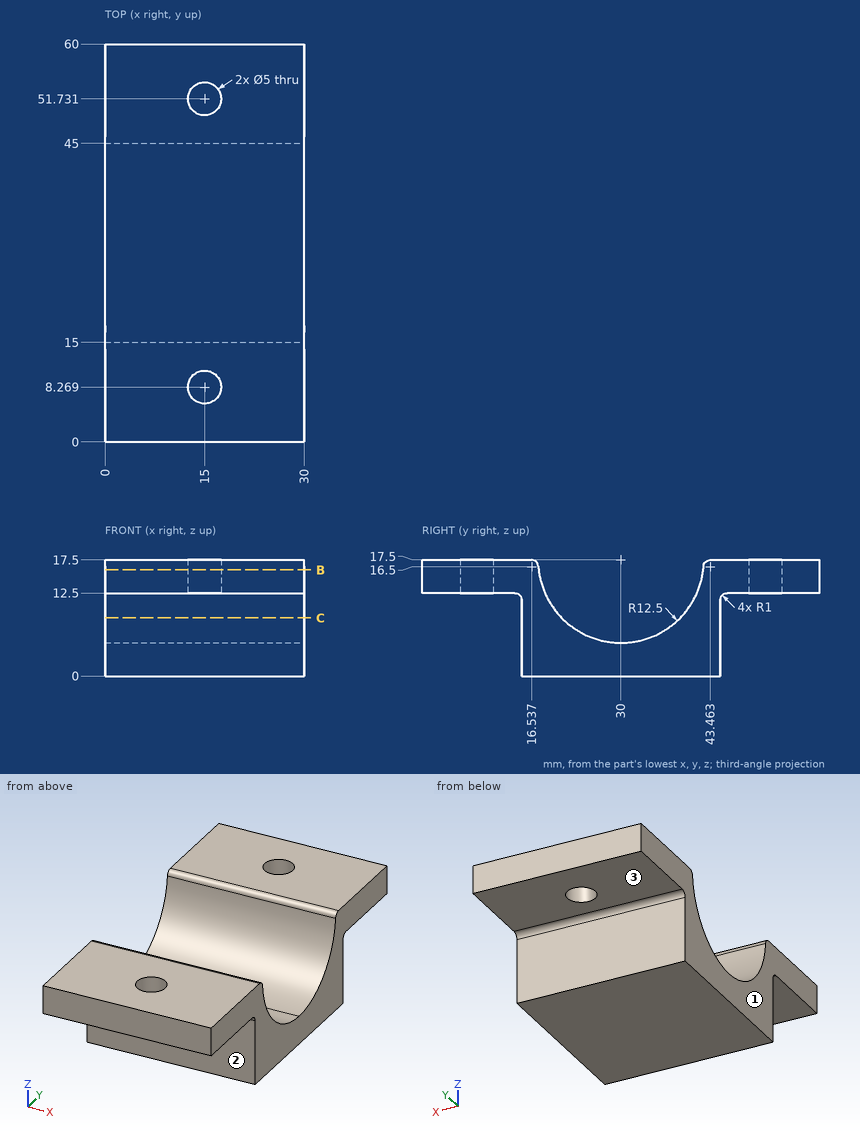
Could you check a few things on this drawing? It's one solid part, dimensions in mm from its lowest x, y, z. A direction names the side the tool comes from. Round coordinates to 2 decimals unless told otherwise and drop trailing zeros. Write each loop counter-clockwise with the first axis right and the second up, starting at its lowest first coordinate (ties: lowest second). Pieces come first, ordered by that corner, then holes. Notation, with made-up numbers: (64.25, -24.75) -> (83.25, -24.75) arc R17 cw to (83.25, -20.75) -> close; hole circle Ø9 at (85.25, 42.25). An arc over 180 degrees is marked (long way). One line per question, with ' | ' between items. Start each with the question number.
1) Suppose I cut it at C-C on z = 8.75. Write out the boundary of the cut face in (x, y).
2) Suppose I cut it at B-B on z = 16. Write out the boundary of the cut face in (x, y), then the cut area to 3 significant figures.
3) I need wall thicknesses on line 1 (Y direction, x = 15, z = 15.85); line 2 (Y direction, x = 15, z = 14.1); line 3 (Y direction, x = 20.75, z = 0.5). Which ranges of each line are inside material? Lowest first, please. Write a range as [from, to].
4) I'm going to push flat-ended pins straight in: P1, Ø8, axis at x = 15, y = 51.73, coming from the -Z side; P2, Ø8, axis at x = 22.5, z = 7, coming from the -Y side; P3, Ø6, axis at x = 13.5, z = 3.5, coming from the +Y side. Where does each tip first touch, or does it pass through?
5) On a 3-axis mill with a long thin cutter (end or side, diameter ignored), from which of +Z, -Z, +X, -X, +Y, -Y can I reach the whole of each face in a straight line? I mean the marked faces 1, 2 and 3. Say none if no direction works.
Return value:
1) outline: (0, 15) -> (30, 15) -> (30, 21.07) -> (0, 21.07) -> close; (0, 38.93) -> (30, 38.93) -> (30, 45) -> (0, 45) -> close
2) outline: (0, 0) -> (30, 0) -> (30, 17.59) -> (0, 17.59) -> close; (0, 42.41) -> (30, 42.41) -> (30, 60) -> (0, 60) -> close; hole circle Ø5 at (15, 8.27); hole circle Ø5 at (15, 51.73) | area: 1,020 mm2
3) line 1: y = [0, 5.77], [10.77, 17.61], [42.39, 49.23], [54.23, 60] | line 2: y = [0, 5.77], [10.77, 17.97], [42.03, 49.23], [54.23, 60] | line 3: y = [15, 45]
4) P1: stops at z = 12.5 | P2: stops at y = 15 | P3: stops at y = 45
5) face 1: +Z, -Z, -X, +Y, -Y | face 2: -Z, +X, -X, -Y | face 3: -Z, +X, -X, +Y
